Check sheet for the drawn part. Datum: minimum x, y, z corner. Units: mm. Coordinates: 2 decimals unless noted, no trailing zeros. Loops run counter-clockwise (first coordinate to the right, second up) from the corner with the lowest first, then second, coordinate; pieces in that order, holes last. Notation, with made-up numbers: (5, 23.25) - (62, 23.25) arc R12 cw to (62, 32.25) - close; hole circle Ø11 at (0, -38). An arc over 180 degrees is marked (long way). Answer as a JSON object with one key per item and string values. Group by question number.
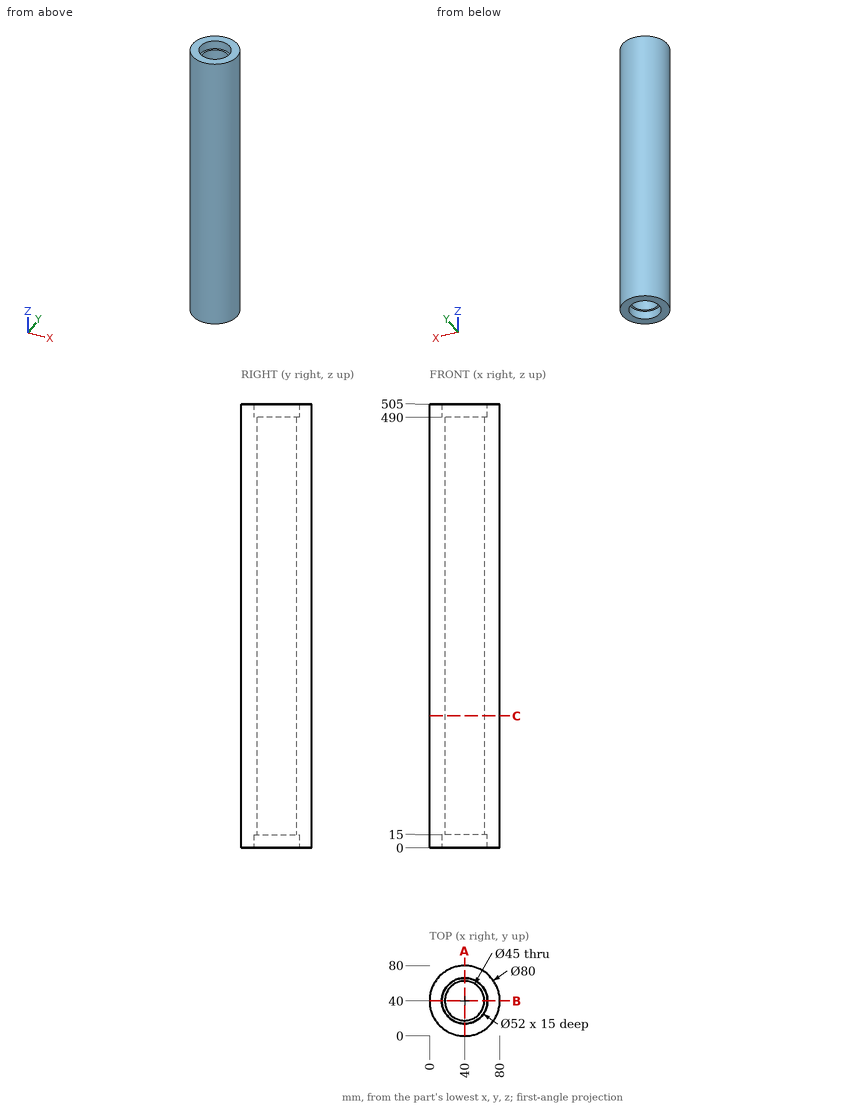
1. Gauge pin test, flat ends, axial feed: pin 1 (10 mm diameter, centred on y = 66.5, z = 258.5, fed in from +X); pin 2 (8 mm diameter, centred on x = 56, y = 67.5, fed in from -Z); pin 3 (6 mm diameter, centred on x = 49, z = 157.5, fed in from +Y); pin 4 (4 mm diameter, centred on y = 64.5, z = 86.5, fed in from -X). Record the tip position at first contact, or that the pin passes through.
2. Sectioned sample at C-C on z = 150. Record the cut outline in (x, y), plus the area to 3 significant figures.
3. Sectioned sample at A-A on x = 40. Record the cut outline in (y, z), plus the area to 3 significant figures.
4. Material ranges on line 1 (Y direction, x = 40, z = 3); line 2 (Y direction, x = 40, z = 351.5); line 3 (Z direction, x = 45.5, y = 63), recorded low to high.
Answers follow:
{
 "1": {"pin 1": "stops at x = 73.73", "pin 2": "stops at z = 0", "pin 3": "stops at y = 79.55", "pin 4": "stops at x = 6.93"},
 "2": {"outline": "circle Ø80 at (40, 40); hole circle Ø45 at (40, 40)", "area": "3,440 mm^2"},
 "3": {"outline": "(0, 0) - (14, 0) - (14, 15) - (17.5, 15) - (17.5, 490) - (14, 490) - (14, 505) - (0, 505) - close; (62.5, 15) - (66, 15) - (66, 0) - (80, 0) - (80, 505) - (66, 505) - (66, 490) - (62.5, 490) - close", "area": "17,500 mm^2"},
 "4": {"line 1": "y = 0 to 14, 66 to 80", "line 2": "y = 0 to 17.5, 62.5 to 80", "line 3": "z = 15 to 490"}
}
